Part model, mm, in its own coordinate system. Face numbers are marked on the shaded views. A direction names the side the tool comes from. Round coordinates to 2 decimals unless told otherwise and drop trailing zeros. Loops run counter-clockwise (first coordinate to the right, second up) from the corner with the lowest first, then second, coordinate; pieces in that order, holes last. Notation, with made-up numbers: (71, -19) -> (103, -19) arc R22 ccw to (103, 19) -> close; hole circle Ø5 at (-37, -32.75). An arc over 180 degrees is marked (long way). Use a Markdown table: item, result. Add a question column.
Item 1: Cut at C-C, the plane z = 0. List the corners of the cut face in (x, y).
Item 2: Cut at D-D, the plane y = 55.5. List the corners of the cut face in (x, z), plus the area to 3 significant figures.
Item 3: Two-plate mould, pull along Z, no slides. Class the marked faces 1, 2 and 3: pulls with the +Z half, pulls with the -Z half, needs draft (parallel to the pull), parting line crosses it, or undercut.
Item 4: Cut at A-A, the plane y = 45.6. List the corners of the cut face in (x, z).
Item 5: Which spindle directions (+Z, -Z, +X, -X, +Y, -Y) get a long thin tool onto all of the face, cutting with end or side? Do the marked faces 4 and 5. Say none if no direction does.
Item 6: Probe line 1 (X direction, y = 10.75, z = 0); line 2 (X direction, y = 18.5, z = 2.5); line 3 (Z direction, x = -43, y = 45). List the from-to ranges inside material, lowest first. Write a range as [from, to].
Item 7: Flat gauge pins, fed straight in: pin 1 (1.5 mm diameter, centred on y = 19.5, z = 2, fed in from +X); pin 2 (3 mm diameter, centred on y = 61.86, z = 16.26, fed in from +X); pin 3 (8 mm diameter, centred on x = 32.64, z = 0, fed in from +Y). Where does each tip first touch, or does it go through?
Item 8: Cut at B-B, the plane z = 10. List the corners of the cut face in (x, y).
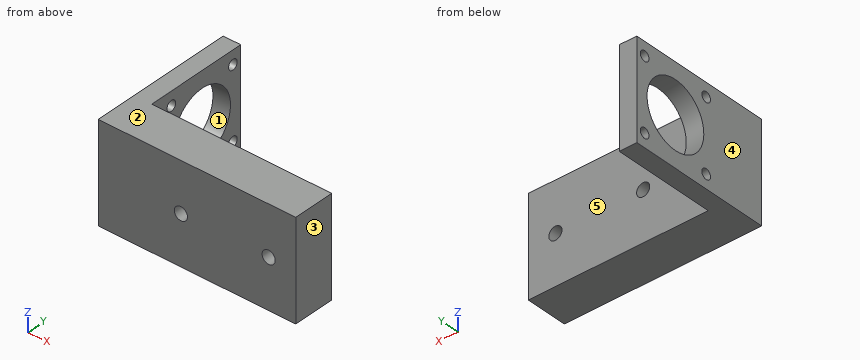
```python
from build123d import *

# Parameters (mm, degrees)
SKETCH1_W           = 90
SKETCH1_H           = 45
BOSS_EXTRUDE1_DEPTH = 5
SKETCH2_W           = 8
SKETCH2_H           = 45
BOSS_EXTRUDE2_DEPTH = 66
SKETCH4_W           = 82
SKETCH4_H           = 45
BOSS_EXTRUDE3_DEPTH = 19
SKETCH5_R           = 15
SKETCH5_R_2         = 2.3
CUT_EXTRUDE1_DEPTH  = 55
SKETCH6_R           = 3
CUT_EXTRUDE2_DEPTH  = 55


with BuildPart() as part:
    # Sketch1 → Boss-Extrude1 (new body)
    with BuildSketch(Plane(origin=(0, 0, 0), x_dir=(1, 0, 0), z_dir=(0, 1, 0))):
        Rectangle(SKETCH1_W, SKETCH1_H)
    extrude(amount=BOSS_EXTRUDE1_DEPTH)

    # Sketch2 → Boss-Extrude2 (add)
    with BuildSketch(Plane(origin=(0, 0, 0), x_dir=(1, 0, 0), z_dir=(0, 1, 0))):
        with Locations((-41, 0)):
            Rectangle(SKETCH2_W, SKETCH2_H)
    extrude(amount=BOSS_EXTRUDE2_DEPTH)

    # Sketch4 → Boss-Extrude3 (add)
    with BuildSketch(Plane(origin=(0, 0, 0), x_dir=(1, 0, 0), z_dir=(0, 1, 0))):
        with Locations((4, 0)):
            Rectangle(SKETCH4_W, SKETCH4_H)
    extrude(amount=BOSS_EXTRUDE3_DEPTH)

    # Sketch5 → Cut-Extrude1 (cut)
    with BuildSketch(Plane(origin=(0, 0, 0), x_dir=(0, 0, -1), z_dir=(1, 0, 0))):
        with Locations((0, 45.6)):
            Circle(SKETCH5_R)
        with Locations((16.263455967, 61.863455967)):
            Circle(SKETCH5_R_2)
        with Locations((16.263455967, 29.336544033)):
            Circle(SKETCH5_R_2)
        with Locations((-16.263455967, 29.336544033)):
            Circle(SKETCH5_R_2)
        with Locations((-16.263455967, 61.863455967)):
            Circle(SKETCH5_R_2)
    extrude(amount=-CUT_EXTRUDE1_DEPTH, mode=Mode.SUBTRACT)

    # Sketch6 → Cut-Extrude2 (cut)
    with BuildSketch(Plane(origin=(0, 0, 0), x_dir=(1, 0, 0), z_dir=(0, 1, 0))):
        with Locations((32.641263943, 0)):
            Circle(SKETCH6_R)
        with Locations((-7.358736057, 0)):
            Circle(SKETCH6_R)
    extrude(amount=CUT_EXTRUDE2_DEPTH, mode=Mode.SUBTRACT)


solid = part.part
```
A:
| question | item | result |
|---|---|---|
| 1 | outline | (-45, 0) -> (-10.36, 0) -> (-10.36, 19) -> (-37, 19) -> (-37, 30.6) -> (-45, 30.6) -> close; (-45, 60.6) -> (-37, 60.6) -> (-37, 66) -> (-45, 66) -> close; (-4.36, 0) -> (29.64, 0) -> (29.64, 19) -> (-4.36, 19) -> close; (35.64, 0) -> (45, 0) -> (45, 19) -> (35.64, 19) -> close |
| 2 | outline | (-45, -22.5) -> (-37, -22.5) -> (-37, -11.27) -> (-45, -11.27) -> close; (-45, 11.27) -> (-37, 11.27) -> (-37, 22.5) -> (-45, 22.5) -> close |
| 2 | area | 180 mm^2 |
| 3 | face 1 | undercut |
| 3 | face 2 | pulls with the +Z half |
| 3 | face 3 | needs draft |
| 4 | outline | (-45, -22.5) -> (-37, -22.5) -> (-37, -15) -> (-45, -15) -> close; (-45, 15) -> (-37, 15) -> (-37, 22.5) -> (-45, 22.5) -> close |
| 5 | face 4 | +Z, -Z, -X, +Y, -Y |
| 5 | face 5 | +Z, -Z, +X, +Y |
| 6 | line 1 | x = [-45, -10.36], [-4.36, 29.64], [35.64, 45] |
| 6 | line 2 | x = [-45, -9.02], [-5.7, 30.98], [34.3, 45] |
| 6 | line 3 | z = [-22.5, -14.99], [14.99, 22.5] |
| 7 | pin 1 | stops at x = 45 |
| 7 | pin 2 | passes through |
| 7 | pin 3 | stops at y = 19 |
| 8 | outline | (-45, 0) -> (45, 0) -> (45, 19) -> (-37, 19) -> (-37, 34.42) -> (-45, 34.42) -> close; (-45, 56.78) -> (-37, 56.78) -> (-37, 66) -> (-45, 66) -> close |
